Autodesk Inventor part; units mm, degrees
ref_plane "YZ Plane" through (0, 0, 0) normal (1, 0, 0) x (0, 1, 0)
ref_plane "XZ Plane" through (0, 0, 0) normal (0, 1, 0) x (-1, 0, 0)
ref_plane "XY Plane" through (0, 0, 0) normal (0, 0, 1) x (1, 0, 0)
sketch "Skizze1" plane through (0, 0, 0) normal (0, 0, 1) x (1, 0, 0)
  line L0 (-220, -220) -> (220, -220)
  line L1 (220, 220) -> (220, -220)
  line L2 (-220, 220) -> (-220, -220)
  line L3 (-220, 220) -> (220, 220)
  line L4 (200, 200) -> (-200, 200)
  line L5 (-200, 200) -> (-200, -200)
  line L6 (-200, -200) -> (200, -200)
  line L7 (200, -200) -> (200, 200)
  line L8 (220, -220) -> (-220, -220)
  line L9 (-220, -220) -> (-220, 220)
  line L10 (-220, 220) -> (220, 220)
  line L11 (220, 220) -> (220, -220)
  line L12 (200, -200) -> (-200, -200)
  line L13 (-200, -200) -> (-200, 200)
  line L14 (-200, 200) -> (200, 200)
  line L15 (200, 200) -> (200, -200)
  point P0 (0, 0)
extrude "Extrusion1" add sketch "Skizze1" against normal blind 20
chamfer "Fase1" distance 20 angle 45 4 edges at (220, 0, -20) (0, 220, -20) (0, -220, -20) (-220, 0, -20)
ref_plane "Arbeitsebene1" through (0, 0, -20) normal (0, 0, 1) x (1, 0, 0)
sketch "Skizze3" plane through (0, 0, -20) normal (0, 0, 1) x (1, 0, 0)
  arc A0 (-205, 25.5) -> (-205, 4.5) centre (-205, 15) ccw
  arc A1 (-205, 25.5) -> (-205, 4.5) centre (-205, 15) ccw
  arc A2 (-205, -5.9522) -> (-205, -26.9522) centre (-205, -16.4522) ccw
  arc A3 (-205, -5.9522) -> (-205, -26.9522) centre (-205, -16.4522) ccw
  arc A4 (-205, -5.9522) -> (-205, -26.9522) centre (-205, -16.4522) ccw
  arc A5 (-205, -5.9522) -> (-205, -26.9522) centre (-205, -16.4522) ccw
  line L0 (-200, -26.9522) -> (-205, -26.9522)
  line L1 (-205, -5.9522) -> (-200, -5.9522)
  line L2 (-205, 4.5) -> (-200, 4.5)
  line L3 (-200, -200) -> (-200, 200)
  line L4 (-205, 25.5) -> (-200, 25.5)
  line L5 (-205, -5.9522) -> (-200, -5.9522)
  line L6 (-205, -26.9522) -> (-200, -26.9522)
  arc A6 (-205, 25.5) -> (-205, 4.5) centre (-205, 15) ccw
  arc A7 (-205, -5.9522) -> (-205, -26.9522) centre (-205, -16.4522) ccw
  point P0 (0, 0)
extrude "Extrusion2" cut sketch "Skizze3" along normal blind 17
sketch "Skizze5" plane through (0, 0, -20) normal (0, 0, 1) x (1, 0, 0)
  line L0 (-200, -26.9522) -> (-200, -200)
  line L1 (-200, -200) -> (200, -200)
  line L2 (200, -200) -> (200, 200)
  line L3 (-200, 200) -> (200, 200)
  line L4 (-200, -200) -> (200, -200)
  line L5 (200, -200) -> (200, 200)
  line L6 (200, 200) -> (-200, 200)
  line L7 (-200, 200) -> (-200, -200)
  line L8 (-190, -190) -> (190, -190)
  line L9 (190, -190) -> (190, 190)
  line L10 (190, 190) -> (-190, 190)
  line L11 (-190, 190) -> (-190, -190)
  point P0 (0, 0)
  dimension "d8" = 10
  dimension "d9" = 10
  dimension "d10" = 10
  dimension "d11" = 10
extrude "Extrusion3" add sketch "Skizze5" along normal blind 10
ref_plane "Arbeitsebene3" through (220, -220, -440) normal (-1, 0, 0) x (0, 0, 1)
sketch "Skizze6" plane through (220, -220, -440) normal (-1, 0, 0) x (0, 0, 1)
  arc A0 (425, 193.0478) -> (425, 214.0478) centre (425, 203.5478) ccw
  arc A1 (425, 224.5) -> (425, 245.5) centre (425, 235) ccw
  line L0 (425, 224.5) -> (420, 224.5)
  line L1 (420, 214.0478) -> (425, 214.0478)
  line L2 (425, 193.0478) -> (420, 193.0478)
  line L3 (420, 245.5) -> (425, 245.5)
  line L4 (420, 193.0478) -> (430, 193.0478)
  line L5 (420, 193.0478) -> (425, 193.0478)
  line L6 (420, 214.0478) -> (425, 214.0478)
  line L7 (430, 214.0478) -> (420, 214.0478)
  line L8 (420, 245.5) -> (420, 224.5)
  line L9 (420, 224.5) -> (425, 224.5)
  line L10 (420, 245.5) -> (425, 245.5)
  line L11 (420, 193.0478) -> (420, 20)
  line L12 (420, 193.0478) -> (420, 214.0478)
  line L13 (420, 224.5) -> (420, 245.5)
  arc A2 (425, 193.0478) -> (425, 214.0478) centre (425, 203.5478) ccw
  arc A3 (425, 224.5) -> (425, 245.5) centre (425, 235) ccw
  point P0 (440, 220)
extrude "Extrusion4" cut sketch "Skizze6" along normal blind 25
properties part number "PV_Ramen_CPY_3_21"
Design review of the part built by this model. Coordinates are the model's own, in mm. A direction names the side the tool comes from. Coordinates: 2 decimals unless noted, no trailing zeros. One line per item, written item: value.
1) Machinability: for faces 1 (the face through (200, -3, -5)), 2 (the face through (205.412, -16.221, -4.503)), 3 (the face through (-190, 3, -15)), 4 (the face through (-215.5, 14.8, -3.8)), which of the approach directions +Z, -Z, +X, -X, +Y, -Y give a long, thin tool a straight path to every point of the face, cutting with its end or side? Answer none if there is none.
Output values:
face 1: +Z
face 2: -Z, +X
face 3: +Z, -Z
face 4: -Z
2) Clearance check with flat-ended pins moving along their axes: P1, Ø5, axis at x = -53, z = -12.5, coming from the -Y side; P2, Ø5, axis at y = -15, z = -17, coming from the -X side; P3, Ø8, axis at y = 83, z = -6.5, coming from the +X side. State where each tip first meets the part, or that it passes through.
Output values:
P1: stops at y = -210
P2: stops at x = -200
P3: stops at x = 217.5
3) To check wall thickness, follow probe 1 along X at (y, z) = (-18, -15.25); probe 2 along X at (y, z) = (-176.5, -9); probe 3 along Z at (x, y) = (-132, -191.5). State the ranges of each line that lie inside material, in increasing order. Write a range as [from, to].
Output values:
probe 1: x = [-200, -190], [190, 195]
probe 2: x = [-211, -200], [200, 211]
probe 3: z = [-20, -10]
